from build123d import *

# Parameters (mm, degrees)
F0_W        = 20
F0_H        = 30
F1_DEPTH    = 20
F0_W_2      = 10
F0_H_2      = 40
F0_W_3      = 40
F0_H_3      = 20
F2_DEPTH    = 5
F3_T        = 2.5
F3_T3_DEPTH = 25
F3_T5_DEPTH = 35
F3_T7_DEPTH = 10


# Not quite as in the source:
# - a shell that OpenCascade refuses in one call is made with other operations: the cavity is built on its own and cut out


with BuildPart() as f1:
    # F0 (on Top) → F1 (new body)
    with BuildSketch(Plane.XY):
        with Locations((71.046166122, 0)):
            Rectangle(F0_W, F0_H)
    extrude(amount=F1_DEPTH)

    # F0 (on Top) → F2 (join)
    with BuildSketch(Plane.XY):
        with BuildLine():
            ThreePointArc((-90, 39.709673646), (-97.1888826467, 35.2686887253), (-100, 27.3))
            Line((-100, 27.3), (-100, 20))
            Line((-100, 20), (-90, 20))
            Line((-90, 20), (-90, 39.709673646))
        make_face()
        with Locations((-95, 0)):
            Rectangle(F0_W_2, F0_H_2)
        with BuildLine():
            Line((-90, -20), (-100, -20))
            Line((-100, -20), (-100, -27.3))
            ThreePointArc((-100, -27.3), (-97.1888826467, -35.2686887253), (-90, -39.709673646))
            Line((-90, -39.709673646), (-90, -20))
        make_face()
        with Locations((-70, 0)):
            Rectangle(F0_W_3, F0_H_2)
        Polygon((-50, 40), (-50, 20), (-50, -20), (-50, -40), (50, -40), (50, -20), (50, 20), (50, 40), align=None)
        with Locations((70, 0)):
            Rectangle(F0_W_3, F0_H_2)
        with Locations((71.046166122, 0)):
            Rectangle(F0_W, F0_H, mode=Mode.SUBTRACT)
        with Locations((95, 0)):
            Rectangle(F0_W_2, F0_H_2)
        with Locations((95, -30)):
            Rectangle(F0_W_2, F0_H_3)
        with Locations((95, 30)):
            Rectangle(F0_W_2, F0_H_3)
    extrude(amount=F2_DEPTH)

    # F3: shell of thickness 2.5, made by hand


with BuildPart() as f3_core1:
    # F3_t2: copy of F1
    add(f1.part)

    # the walls: a layer under each face that stays
    f3_faces = [f3_core1.faces().sort_by_distance(p)[0] for p in [
        (71.046166122, 15, 12.5),
        (0, 0, 5),
        (61.046166122, 0, 12.5),
        (71.046166122, 0, 20),
        (81.046166122, 0, 12.5),
        (-97.1888826467, 35.2686887253, 2.5),
        (-100, 0, 2.5),
        (-97.1888826467, -35.2686887253, 2.5),
        (-90, -29.854836823, 2.5),
        (-70, -20, 2.5),
        (-50, -30, 2.5),
        (0, -40, 2.5),
        (50, -30, 2.5),
        (70, -20, 2.5),
        (90, -30, 2.5),
        (95, -40, 2.5),
        (100, 0, 2.5),
        (95, 40, 2.5),
        (90, 30, 2.5),
        (70, 20, 2.5),
        (50, 30, 2.5),
        (0, 40, 2.5),
        (-50, 30, 2.5),
        (-70, 20, 2.5),
        (-90, 29.854836823, 2.5),
        (0, 0, 0),
    ]]
    thicken(f3_faces, amount=-F3_T, mode=Mode.SUBTRACT)

    # F3_s4 → F3_t3 (cut)
    with BuildSketch(Plane.YZ.offset(58.546166122)):
        Polygon((15.025, 5.025), (12.5, 5), (12.5, 2.5), (15, 2.5), align=None)
    extrude(amount=F3_T3_DEPTH, mode=Mode.SUBTRACT)

    # F3_s6 → F3_t5 (cut)
    with BuildSketch(Plane.XZ.offset(-17.5)):
        Polygon((61.021166122, 5.025), (61.046166122, 2.5), (63.546166122, 2.5), (63.546166122, 5), align=None)
        Polygon((81.071166122, 5.025), (81.046166122, 2.5), (78.546166122, 2.5), (78.546166122, 5), align=None)
    extrude(amount=F3_T5_DEPTH, mode=Mode.SUBTRACT)

    # F3_s8 → F3_t7 (cut)
    with BuildSketch(Plane.XY.offset(-2.5)):
        Polygon((-89.975, -20.025), (-92.5, -20), (-92.5, -17.5), (-90, -17.5), align=None)
        Polygon((-50.025, -20.025), (-50, -17.5), (-47.5, -17.5), (-47.5, -20), align=None)
        Polygon((50.025, -20.025), (47.5, -20), (47.5, -17.5), (50, -17.5), align=None)
        Polygon((89.975, -20.025), (90, -17.5), (92.5, -17.5), (92.5, -20), align=None)
        Polygon((89.975, 20.025), (92.5, 20), (92.5, 17.5), (90, 17.5), align=None)
        Polygon((50.025, 20.025), (50, 17.5), (47.5, 17.5), (47.5, 20), align=None)
        Polygon((-50.025, 20.025), (-47.5, 20), (-47.5, 17.5), (-50, 17.5), align=None)
        Polygon((-89.975, 20.025), (-90, 17.5), (-92.5, 17.5), (-92.5, 20), align=None)
    extrude(amount=F3_T7_DEPTH, mode=Mode.SUBTRACT)


with BuildPart() as f1_1:
    add(f1.part)

    # what is left inside the walls is the cavity
    f3_cavity = [f3_core1.part.solids().sort_by_distance(p)[0] for p in [
        (71.046166, -5.833333, 17.475),
    ]]
    add(f3_cavity, mode=Mode.SUBTRACT)


solid = f1_1.part
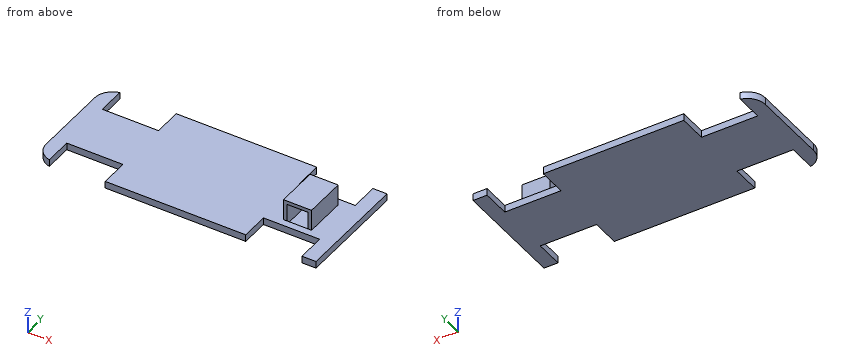
Geometry check sheet. Reference: the model listing, model coordinates, mm. Give positions to 0.01 mm unless a question says otherwise; leave off trailing zeros. Write each loop counter-clockwise with the first axis right and the second up, starting at its lowest first coordinate (ties: lowest second). Pieces come first, ordered by that corner, then holes. Notation, with made-up numbers: (44.5, -5.5) - (94.5, -5.5) arc R19 cw to (94.5, 30.5) - close; hole circle Ø3 at (-26.5, 17.25). An arc over 180 degrees is marked (long way). Put each result on its own line as item: value.
1. Thickness scan on line 1 (X direction, y = 26, z = 1.5); line 2 (X direction, y = -14, z = 9); line 3 (Y direction, x = 66.5, z = 4.5). Record the ranges inside material, lowest first.
Ans:
line 1: x = -100 to -90, -50 to 50, 90 to 100
line 2: x = 61.05 to 63.55, 78.55 to 81.05
line 3: y = -20 to -15, 12.5 to 20
2. Sectioned sample at B-B, the plane x = 70. Enter the section's corners in (y, z), plus the area to 4 significant figures.
Ans:
outline: (-20, 0) - (20, 0) - (20, 5) - (15, 5) - (15, 20) - (-15, 20) - (-15, 17.5) - (12.5, 17.5) - (12.5, 2.5) - (-15, 2.5) - (-15, 5) - (-20, 5) - close
area: 237.5 mm²
3. Sectioned sample at A-A, the plane y = -4. Enter the section's corners in (x, z), plus the area to 4 significant figures.
Ans:
outline: (-100, 0) - (100, 0) - (100, 5) - (81.05, 5) - (81.05, 20) - (61.05, 20) - (61.05, 5) - (-100, 5) - close; hole (63.55, 2.5) - (78.55, 2.5) - (78.55, 17.5) - (63.55, 17.5) - close
area: 1,075 mm²
4. Sectioned sample at D-D, the plane y = -32. Enter the section's corners in (x, z), plus the area to 3 significant figures.
Ans:
outline: (-99.1, 0) - (-90, 0) - (-90, 5) - (-99.1, 5) - close; (-50, 0) - (50, 0) - (50, 5) - (-50, 5) - close; (90, 0) - (100, 0) - (100, 5) - (90, 5) - close
area: 595 mm²
5. Sectioned sample at C-C, the plane z = 14.5. Enter the section's corners in (x, y), plus the area to 4 significant figures.
Ans:
outline: (61.05, -15) - (63.55, -15) - (63.55, 12.5) - (78.55, 12.5) - (78.55, -15) - (81.05, -15) - (81.05, 15) - (61.05, 15) - close
area: 187.5 mm²
6. Go/stop test with flat-tipped pins: pin 1 (1.5 mm diameter, centred on x = -77.5, z = 3.5, fed in from -Y); pin 2 (4 mm diameter, centred on x = -40.5, z = 7.5, fed in from +Y); pin 3 (4.5 mm diameter, centred on x = 73, z = 10.5, fed in from +Y); pin 4 (0.8 mm diameter, centred on x = 69.5, z = 4, fed in from +Y). Record where each tip stops, or that it passes through.
Ans:
pin 1: stops at y = -20
pin 2: passes through
pin 3: stops at y = 15
pin 4: stops at y = 20
